Design review of the part built by this model. Coordinates are the model's own, in mm. Face numbers are marked on the shaded views. Give positions to 0.01 mm unless a question says otherwise; leave off trailing zeros. Order: outer loops, then holes, each group sorted by start corner. A loop starts at its lowest first (then second) coordinate and runs counter-clockwise, first axis right, second up.
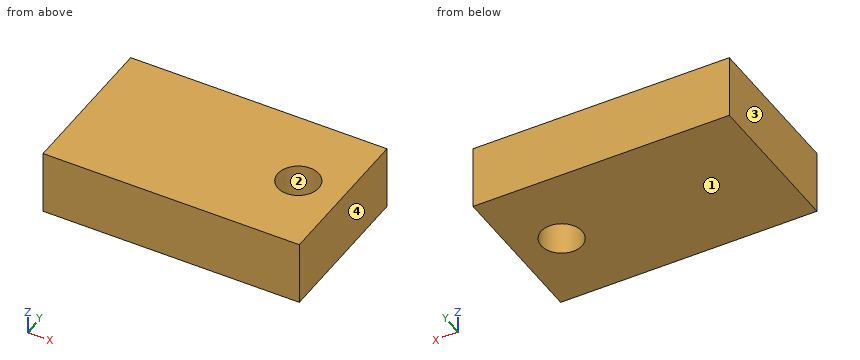
```python
from build123d import *

# Parameters (mm, degrees)
F0_R     = 1.6
F1_DEPTH = 5


with BuildPart() as f1:
    # F0 (on Top) → F1 (new body)
    with BuildSketch(Plane.XY):
        with Locations((6.5, 0)):
            Circle(F0_R)
        Polygon((10, 0), (10, 6), (-10, 6), (-10, -6), (10, -6), align=None)
        with Locations((6.5, 0)):
            Circle(F0_R, mode=Mode.SUBTRACT)
    extrude(amount=F1_DEPTH)


solid = f1.part
```
1. Take a section at A-A (x = 6.5). State the section outline as (y, z) points.
Recorded:
outline: (-6, 0) - (-1.6, 0) - (-1.6, 5) - (-6, 5) - close; (1.6, 0) - (6, 0) - (6, 5) - (1.6, 5) - close
2. Take a section at B-B (y = 0). State the section outline as (x, z) points.
Recorded:
outline: (-10, 0) - (4.9, 0) - (4.9, 5) - (-10, 5) - close; (8.1, 0) - (10, 0) - (10, 5) - (8.1, 5) - close
3. For line 1 along Y through (x, z) = (6.5, 1.7); line 2 along Y through (x, z) = (5.25, 0.8); line 3 along X through (y, z) = (1.25, 0.95), list the stretches that pass through material, from the lowest coordinate up.
Recorded:
line 1: y = -6 to -1.6, 1.6 to 6
line 2: y = -6 to -1, 1 to 6
line 3: x = -10 to 5.5, 7.5 to 10
4. Draft analysis for pull direction X (two halves, no side actions). For the marked faces 1, 2, 3 and 4, state which applies: pulls with the +X half, pulls with the -X half, needs draft (parallel to the pull), parting line crosses it, or undercut.
Recorded:
face 1: needs draft
face 2: undercut
face 3: pulls with the -X half
face 4: pulls with the +X half
5. Take a section at C-C (z = 0.75). State the section outline as (x, y) points, then the cut area to 3 significant figures.
Recorded:
outline: (-10, -6) - (10, -6) - (10, 6) - (-10, 6) - close; hole circle Ø3.2 at (6.5, 0)
area: 232 mm2
6. For pin 1 (3 mm diameter, centred on x = 6.5, y = 0, fed in from -Z), flat-tipped, find the tip position at first contact; note if it passes through.
Recorded:
pin 1: passes through
